from build123d import *

# Parameters (mm, degrees)
SKETCH_1_R           = 40
EXTRUDE_1_DEPTH      = 59
CUT_EXTRUDE_1_DEPTH  = 5
SKETCH_4_R           = 9
CUT_EXTRUDE_2_DEPTH  = 108.14942837
CUT_EXTRUDE_START    = -2
SKETCH_7_R           = 40
SKETCH_7_R_2         = 37
CUT_EXTRUDE_4_DEPTH  = 2
SKETCH_8_R           = 40
SKETCH_8_R_2         = 37
CUT_EXTRUDE_5_DEPTH  = 2
CUT_EXTRUDE_START_2  = -3
SKETCH_10_R          = 40
SKETCH_10_R_2        = 37
CUT_EXTRUDE_6_DEPTH  = 3
SKETCH_6_R           = 30
CUT_EXTRUDE_7_DEPTH  = 6
FILLET_2_R           = 5
SKETCH_17_R          = 10
CUT_EXTRUDE_11_DEPTH = 0.5
SKETCH_13_R          = 27
CUT_EXTRUDE_12_DEPTH = 46.5
EXTRUDE_2_DEPTH      = 19
SKETCH_21_R          = 9
CUT_EXTRUDE_13_DEPTH = 108.149428483
SKETCH_22_R          = 9
CUT_EXTRUDE_14_DEPTH = 89.82567207
FILLET_7_R           = 5


with BuildPart() as part:
    # Sketch 1 → Extrude 1 (new body)
    with BuildSketch(Plane(origin=(0, 0, 0), x_dir=(1, 0, 0), z_dir=(0, 1, 0))):
        with Locations(Location((0, 0, 0), (0, 0, 270))):
            Circle(SKETCH_1_R)
    extrude(amount=EXTRUDE_1_DEPTH)

    # Sketch 2 → Cut-Extrude 1 (cut)
    with BuildSketch(Plane(origin=(0, 0, 0), x_dir=(-1, 0, 0), z_dir=(0, -1, 0))):
        with BuildLine():
            Line((-19.364916731, -35), (19.364916731, -35))
            ThreePointArc((19.364916731, -35), (40, 0), (19.364916731, 35))
            Line((19.364916731, 35), (-19.364916731, 35))
            ThreePointArc((-19.364916731, 35), (-40, 0), (-19.364916731, -35))
        make_face()
    extrude(amount=-CUT_EXTRUDE_1_DEPTH, mode=Mode.SUBTRACT)

    # Sketch 4 → Cut-Extrude 2 (cut, through all)
    with BuildSketch(Plane(origin=(40, 0, 0), x_dir=(0, 0, -1), z_dir=(1, 0, 0))):
        with Locations((0, 25)):
            Circle(SKETCH_4_R)
    cut_extrude_2 = extrude(amount=-CUT_EXTRUDE_2_DEPTH, mode=Mode.SUBTRACT)

    # Sketch 7 → Cut-Extrude 4 (cut)
    with BuildSketch(Plane(origin=(0, 53, 0), x_dir=(1, 0, 0), z_dir=(0, 1, 0)).offset(CUT_EXTRUDE_START)):
        with Locations(Location((0, 0, 0), (0, 0, 61.044975628))):
            Circle(SKETCH_7_R)
        with Locations(Location((0, 0, 0), (0, 0, 270))):
            Circle(SKETCH_7_R_2, mode=Mode.SUBTRACT)
    extrude(amount=CUT_EXTRUDE_4_DEPTH, mode=Mode.SUBTRACT)

    # Sketch 8 → Cut-Extrude 5 (cut)
    with BuildSketch(Plane(origin=(0, 48, 0), x_dir=(1, 0, 0), z_dir=(0, 1, 0)).offset(CUT_EXTRUDE_START)):
        with Locations(Location((0, 0, 0), (0, 0, 270))):
            Circle(SKETCH_8_R)
        with Locations(Location((0, 0, 0), (0, 0, 270))):
            Circle(SKETCH_8_R_2, mode=Mode.SUBTRACT)
    extrude(amount=CUT_EXTRUDE_5_DEPTH, mode=Mode.SUBTRACT)

    # Sketch 10 → Cut-Extrude 6 (cut)
    with BuildSketch(Plane(origin=(0, 44, 0), x_dir=(1, 0, 0), z_dir=(0, 1, 0)).offset(CUT_EXTRUDE_START_2)):
        with Locations(Location((0, 0, 0), (0, 0, 270))):
            Circle(SKETCH_10_R)
        with Locations(Location((0, 0, 0), (0, 0, 270))):
            Circle(SKETCH_10_R_2, mode=Mode.SUBTRACT)
    extrude(amount=CUT_EXTRUDE_6_DEPTH, mode=Mode.SUBTRACT)

    # Sketch 6 → Cut-Extrude 7 (cut)
    with BuildSketch(Plane(origin=(0, 59, 0), x_dir=(1, 0, 0), z_dir=(0, 1, 0))):
        with Locations(Location((0, 0, 0), (0, 0, 270))):
            Circle(SKETCH_6_R)
    extrude(amount=-CUT_EXTRUDE_7_DEPTH, mode=Mode.SUBTRACT)

    # Fillet 2
    fillet_2_edges = [part.edges().sort_by_distance(p)[0] for p in [
        (0, 53, -30),
    ]]
    fillet(fillet_2_edges, radius=FILLET_2_R)

    # Sketch 17 → Cut-Extrude 11 (cut)
    with BuildSketch(Plane(origin=(38, 0, 0), x_dir=(0, 0, -1), z_dir=(1, 0, 0))):
        with Locations((0, 25)):
            Circle(SKETCH_17_R)
    cut_extrude_11 = extrude(amount=CUT_EXTRUDE_11_DEPTH, mode=Mode.SUBTRACT)

    # Mirror 1: Cut-Extrude 11 across plane
    add(cut_extrude_11.mirror(Plane(origin=(0, 0, 0), x_dir=(0, 0, 1), z_dir=(1, 0, 0))), mode=Mode.SUBTRACT)

    # Mirror 1 at the second plane: Cut-Extrude 11 across plane
    add(cut_extrude_11.mirror(Plane.XY), mode=Mode.SUBTRACT)

    # Sketch 13 → Cut-Extrude 12 (cut)
    with BuildSketch(Plane(origin=(0, 0, 0), x_dir=(1, 0, 0), z_dir=(0, 1, 0))):
        with Locations(Location((0, 0, 0), (0, 0, 90))):
            Circle(SKETCH_13_R)
    extrude(amount=CUT_EXTRUDE_12_DEPTH, mode=Mode.SUBTRACT)

    # Sketch 16 → Extrude 2 (add)
    with BuildSketch(Plane(origin=(13, 0, 0), x_dir=(0, 0, -1), z_dir=(1, 0, 0))):
        with BuildLine():
            Line((-13, 25), (-13, 46.5))
            Line((-13, 46.5), (13, 46.5))
            Line((13, 46.5), (13, 25))
            ThreePointArc((13, 25), (0, 12), (-13, 25))
        make_face()
    extrude_2 = extrude(amount=EXTRUDE_2_DEPTH)

    # Sketch 21 → Cut-Extrude 13 (cut, through all)
    with BuildSketch(Plane(origin=(40, 0, 0), x_dir=(0, 0, -1), z_dir=(1, 0, 0))):
        with Locations((0, 25)):
            Circle(SKETCH_21_R)
    extrude(amount=-CUT_EXTRUDE_13_DEPTH, mode=Mode.SUBTRACT)

    # Mirror 2: Extrude 2 across plane
    add(extrude_2.mirror(Plane(origin=(0, 0, 0), x_dir=(0, 0, 1), z_dir=(1, 0, 0))))

    # Sketch 22 → Cut-Extrude 14 (cut, through all)
    with BuildSketch(Plane(origin=(13, 0, 0), x_dir=(0, 0, -1), z_dir=(1, 0, 0))):
        with Locations((0, 24.451782415)):
            Circle(SKETCH_22_R)
    extrude(amount=CUT_EXTRUDE_14_DEPTH, mode=Mode.SUBTRACT)

    # Mirror 3: Cut-Extrude 2 across plane
    add(cut_extrude_2.mirror(Plane(origin=(0, 0, 0), x_dir=(0, 0, 1), z_dir=(1, 0, 0))), mode=Mode.SUBTRACT)

    # Fillet 7
    fillet_7_edges = [part.edges().sort_by_distance(p)[0] for p in [
        (0, 46.5, 27),
        (13.747727085, 46.5, -23.237900077),
    ]]
    fillet(fillet_7_edges, radius=FILLET_7_R)


solid = part.part
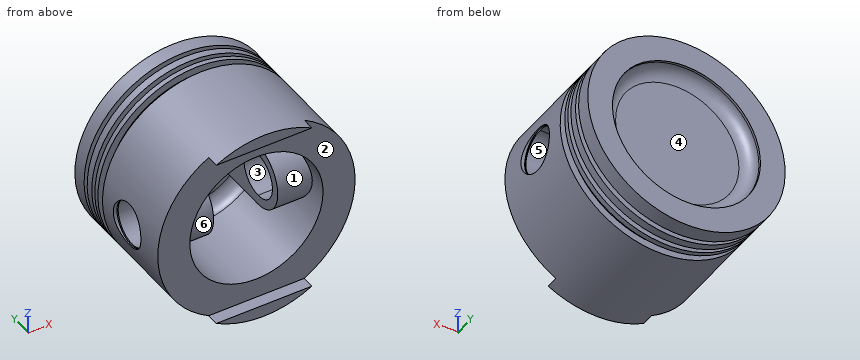
Input: part model. Units: mm. Frame: model coordinates. Face numbers are marked on the shaded views. A direction names the side the tool comes from. Round coordinates to 2 decimals unless told otherwise and drop trailing zeros. Order: outer loops, then holes, each group sorted by start corner. A loop starts at its lowest first (then second) coordinate and runs counter-clockwise, first axis right, second up. Notation, with made-up numbers: (23.5, -24) - (82.5, -24) arc R26 ccw to (82.5, 6) - close; hole circle Ø7 at (-29, 66). An arc over 180 degrees is marked (long way). Answer as a JSON object with one key per item and string values. Group by question number.
(1) Cut plane D-D (y = 9.5). Return loops of the section in (x, z), then the cut area to 3 significant figures.
(2) Draft query along Y for the marked faces 4, 5 and 6. Return one class per face: released by +Y, released by -Y, zero draft, split by the parting line, or undercut.
(3) Material intervals for probe 1 along Y at (x, z) = (38.25, 0); probe 2 along Y at (x, z) = (-34.5, -19.5); probe 3 along Z at (x, y) = (-21.5, 39), sorted ascending. Write a range as from..to.
(4) Reachability of the marked faces 1, 2 and 3 from +Z, -Z, +X, -X, +Y, -Y: full face, straight path, thin tool, end or side. Return the list, or none.
(5) Cut plane C-C (z = 0). Count the separate pieces of the cut face and the enclosed holes in it, then the cut area to 3 significant figures.
(6) Pin query (flat end, axial travel): P1, Ø22, axis at y = 24.5, z = 1, coming from the -X side; P2, Ø10, axis at y = 50, z = 8.5, coming from the +X side; P3, Ø3, axis at x = -18, y = 34, coming from the +Z side; P4, Ø11, axis at y = 25, z = 0, coming from the +X side. Return the tip coordinate at first contact, or that it passes through.
Here are the results:
{
 "1": {"outline": "circle Ø80 at (0, 0); hole circle Ø54 at (0, 0)", "area": "2,740 mm^2"},
 "2": {"face 4": "released by +Y", "face 5": "undercut", "face 6": "released by -Y"},
 "3": {"probe 1": "y = 5..15, 35..41, 44..46, 48..51, 53..59", "probe 2": "y = 5..41, 44..46, 48..51, 53..59", "probe 3": "z = -33.73..-16.33, -13..13, 16.33..33.73"},
 "4": {"face 1": "-Y", "face 2": "+X, -X, -Y", "face 3": "+X, -X"},
 "5": {"separate pieces": "3", "enclosed holes": "0", "area": "1,670 mm^2"},
 "6": {"P1": "stops at x = -40", "P2": "stops at x = 39.85", "P3": "stops at z = 36.44", "P4": "passes through"}
}
